Read the model definition and answer for the solid it produces. Units are mm, in the model's axes. A direction names the side the tool comes from. Coordinates: 2 decimals unless noted, no trailing zeros. Loops run counter-clockwise (first coordinate to the right, second up) from the corner with the lowest first, then second, coordinate; pieces in that order, holes last. Notation, with made-up numbers: (2, 86) - (17, 86) arc R25 ccw to (17, 116) - close; hole circle Ø4 at (78.25, -22). An arc over 180 degrees is marked (long way). One line per item, written item: value. Start each with the question number.
from build123d import *

# Parameters (mm, degrees)
SKETCH_1_W          = 76
SKETCH_1_H          = 23.8
SKETCH_1_R          = 1.9
EXTRUDE_1_DEPTH     = 3
SKETCH_3_W          = 76
SKETCH_3_H          = 3
EXTRUDE_2_DEPTH     = 10
SKETCH_4_R          = 1.6
CUT_EXTRUDE_1_DEPTH = 10
SKETCH_5_W          = 60
SKETCH_5_H          = 7.8
CUT_EXTRUDE_2_DEPTH = 10
SKETCH_6_R          = 1.6
SKETCH_6_W          = 76
SKETCH_6_H          = 25
SKETCH_6_R_2        = 1.9
SKETCH_6_W_2        = 60
SKETCH_6_H_2        = 7.8
EXTRUDE_3_DEPTH     = 3


with BuildPart() as part:
    # Sketch 1 → Extrude 1 (new body)
    with BuildSketch(Plane(origin=(0, 0, 0), x_dir=(1, 0, 0), z_dir=(0, 1, 0))):
        with Locations((33, -6.9)):
            Rectangle(SKETCH_1_W, SKETCH_1_H)
        with Locations(Location((0, 0, 0), (0, 0, 270))):
            Circle(SKETCH_1_R, mode=Mode.SUBTRACT)
        with Locations(Location((0, -13.8, 0), (0, 0, 270))):
            Circle(SKETCH_1_R, mode=Mode.SUBTRACT)
        with Locations(Location((66, 0, 0), (0, 0, 270))):
            Circle(SKETCH_1_R, mode=Mode.SUBTRACT)
        with Locations(Location((66, -13.8, 0), (0, 0, 270))):
            Circle(SKETCH_1_R, mode=Mode.SUBTRACT)
    extrude(amount=EXTRUDE_1_DEPTH)

    # Sketch 3 → Extrude 2 (add)
    with BuildSketch(Plane(origin=(0, 0, -5), x_dir=(-1, 0, 0), z_dir=(0, 0, -1))):
        with Locations((-33, 1.5)):
            Rectangle(SKETCH_3_W, SKETCH_3_H)
    extrude(amount=EXTRUDE_2_DEPTH)

    # Sketch 4 → Cut-Extrude 1 (cut)
    with BuildSketch(Plane(origin=(0, 3, 0), x_dir=(1, 0, 0), z_dir=(0, 1, 0))):
        with Locations(Location((3, 10, 0), (0, 0, 270))):
            Circle(SKETCH_4_R)
        with Locations(Location((33, 10, 0), (0, 0, 270))):
            Circle(SKETCH_4_R)
        with Locations(Location((63, 10, 0), (0, 0, 270))):
            Circle(SKETCH_4_R)
    extrude(amount=-CUT_EXTRUDE_1_DEPTH, mode=Mode.SUBTRACT)

    # Sketch 5 → Cut-Extrude 2 (cut)
    with BuildSketch(Plane(origin=(0, 3, 0), x_dir=(1, 0, 0), z_dir=(0, 1, 0))):
        with Locations((33, -6.9)):
            Rectangle(SKETCH_5_W, SKETCH_5_H)
    extrude(amount=-CUT_EXTRUDE_2_DEPTH, mode=Mode.SUBTRACT)

    # Sketch 6 → Extrude 3 (add)
    # profile 1 of 4: a face of its own
    with BuildSketch(Plane(origin=(0, 3, 0), x_dir=(1, 0, 0), z_dir=(0, 1, 0))):
        with Locations(Location((63, 10, 0), (0, 0, 270))):
            Circle(SKETCH_6_R)
    # profile 2 of 4: a face of its own
    with BuildSketch(Plane(origin=(0, 3, 0), x_dir=(1, 0, 0), z_dir=(0, 1, 0))):
        with Locations(Location((33, 10, 0), (0, 0, 270))):
            Circle(SKETCH_6_R)
    # profile 3 of 4: a face of its own
    with BuildSketch(Plane(origin=(0, 3, 0), x_dir=(1, 0, 0), z_dir=(0, 1, 0))):
        with Locations(Location((3, 10, 0), (0, 0, 270))):
            Circle(SKETCH_6_R)
    # profile 4 of 4: a face of its own
    with BuildSketch(Plane(origin=(0, 3, 0), x_dir=(1, 0, 0), z_dir=(0, 1, 0))):
        with Locations((33, -6.3)):
            Rectangle(SKETCH_6_W, SKETCH_6_H)
        with Locations(Location((66, -13.8, 0), (0, 0, 270))):
            Circle(SKETCH_6_R_2, mode=Mode.SUBTRACT)
        with Locations(Location((66, 0, 0), (0, 0, 270))):
            Circle(SKETCH_6_R_2, mode=Mode.SUBTRACT)
        with Locations(Location((0, -13.8, 0), (0, 0, 270))):
            Circle(SKETCH_6_R_2, mode=Mode.SUBTRACT)
        with Locations(Location((0, 0, 0), (0, 0, 270))):
            Circle(SKETCH_6_R_2, mode=Mode.SUBTRACT)
        with Locations((33, -6.9)):
            Rectangle(SKETCH_6_W_2, SKETCH_6_H_2, mode=Mode.SUBTRACT)
    extrude(amount=EXTRUDE_3_DEPTH)


with BuildPart() as extrude_3_kept_piece:
    # of the separate pieces the step leaves, the one the design keeps (extrude_3_pieces_kept)
    add(part.part.solids().sort_by_distance((-5, 0, 18.8))[0])


solid = extrude_3_kept_piece.part
1) For faces 5 (the flat face through (34, 3, -12)), 6 (the flat face through (32, 3, 18.8)), 7 (the flat face through (3, 3, 7)), determine the directions among +Z, -Z, +X, -X, +Y, -Y from which every point of the face is accessible in a straight line to the end or side of a thin tool.
2) Determine the mould class of faces 1 (the cylindrical face through (3.07, 1.52, -11.6)), 2 (the flat face through (-5, 3, 2)), 3 (the flat face through (33, 3, 3)), 4 (the flat face through (32, 4, -6.2)) for opening direction X: released by +X, released by -X, zero draft, split by the parting line, or undercut.
3) Section B-B, the plane z = 9.5 is taken. Determine the outline of the cut face in (x, y), and give its area (3 significant figures).
4) Section A-A, the plane x = 33 is taken. Determine the outline of the cut face in (y, z).
5) Straight lines are drawn through the part: L1, parallel to X at y = 1.45, z = -10; L2, parallel to X at y = 2.7, z = 0; L3, parallel to Z at x = 52, y = 3.1. For each, find the intervals that lie inside material, in ascending order.
6) Section D-D, the plane z = 13.8 is taken. Determine the outline of the cut face in (x, y), and give its area (3 significant figures).
7) Flat-ended cylindrical pins translate along their axes: P1, Ø1.5, axis at x = 45, y = 5, coming from the -Z side; P2, Ø4.5, axis at x = 19.5, z = -11, coming from the +Y side; P3, Ø2.5, axis at x = 33, z = -10, coming from the +Y side. Find the tip coordinate at first contact, or state that the pin passes through.
8) Section C-C, the plane y = 2.1 is taken. State how many separate pieces and enclosed holes the cut face has, and give its area (3 significant figures).
Answer below:
1. face 5: -Z, +X, -X, +Y
1. face 6: +Z, +X, -X, +Y, -Y
1. face 7: +Y, -Y
2. face 1: undercut
2. face 2: released by -X
2. face 3: undercut
2. face 4: zero draft
3. outline: (-5, 0) - (3, 0) - (3, 6) - (-5, 6) - close; (63, 0) - (71, 0) - (71, 6) - (63, 6) - close
3. area: 96.0 mm2
4. outline: (0, -15) - (3, -15) - (3, -11.6) - (0, -11.6) - close; (0, -8.4) - (3, -8.4) - (3, -6.2) - (6, -6.2) - (6, 3) - (0, 3) - close; (0, 10.8) - (6, 10.8) - (6, 18.8) - (0, 18.8) - close
5. L1: -5 to 1.4, 4.6 to 31.4, 34.6 to 61.4, 64.6 to 71
5. L2: -5 to -1.9, 1.9 to 64.1, 67.9 to 71
5. L3: -6.2 to 3, 10.8 to 18.8
6. outline: (-5, 0) - (-1.9, 0) - (-1.9, 6) - (-5, 6) - close; (1.9, 0) - (64.1, 0) - (64.1, 6) - (1.9, 6) - close; (67.9, 0) - (71, 0) - (71, 6) - (67.9, 6) - close
6. area: 410 mm2
7. P1: z = -6.2
7. P2: y = 3
7. P3: through
8. separate pieces: 1
8. enclosed holes: 8
8. area: 2,030 mm2
